Build history of the part. All positions in model axes, mm. Round coordinates to 2 decimals unless told otherwise and drop trailing zeros. Loops run counter-clockwise (first coordinate to the right, second up) from the corner with the lowest first, then second, coordinate; pieces in that order, holes last. Notation, with made-up numbers: M -23,89.25 L -4,89.25 A33 ccw -4,125.25 Z; hole C -9,-7.75 d10. An arc over 180 degrees is marked long. One line per item, written item: value.
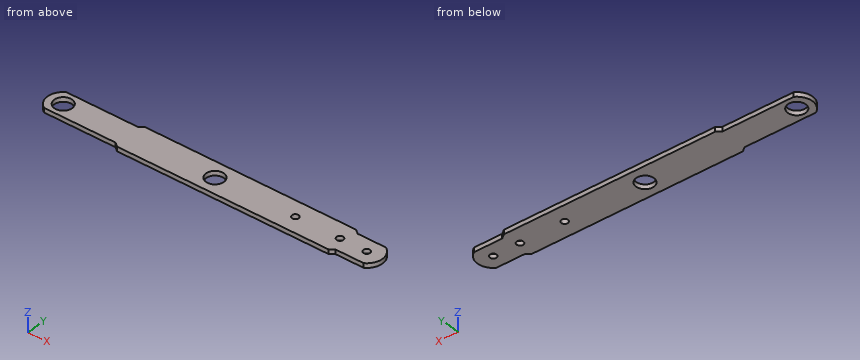
```python
from build123d import *

# Parameters (mm, degrees)
ESQUISSE1_R      = 1.5
ESQUISSE1_R_2    = 4
EXTRUSION1_DEPTH = 2


with BuildPart() as part:
    # Esquisse1 → Extrusion1 (new body)
    with BuildSketch(Plane.XY):
        with BuildLine():
            Line((71.605551275, 6), (59, 6))
            Line((59, 6), (57, 7.5))
            Line((57, 7.5), (-37.605551275, 7.5))
            Line((-37.605551275, 7.5), (-39.605551275, 6))
            Line((-39.605551275, 6), (-71.605551275, 6))
            ThreePointArc((-71.605551275, 6), (-75, 0), (-71.605551275, -6))
            Line((-71.605551275, -6), (-39.605551275, -6))
            Line((-39.605551275, -6), (-37.605551275, -7.5))
            Line((-37.605551275, -7.5), (57, -7.5))
            Line((57, -7.5), (59, -6))
            Line((59, -6), (71.605551275, -6))
            ThreePointArc((71.605551275, -6), (75, 0), (71.605551275, 6))
        make_face()
        with Locations((68, 0)):
            Circle(ESQUISSE1_R, mode=Mode.SUBTRACT)
        with Locations(Location((-68, 0, 0), (0, 0, 180))):
            Circle(ESQUISSE1_R_2, mode=Mode.SUBTRACT)
        Circle(ESQUISSE1_R_2, mode=Mode.SUBTRACT)
        with Locations((56, 0)):
            Circle(ESQUISSE1_R, mode=Mode.SUBTRACT)
        with Locations((36, 0)):
            Circle(ESQUISSE1_R, mode=Mode.SUBTRACT)
    extrude(amount=EXTRUSION1_DEPTH)


solid = part.part
```
Item 1: Drop flat-ended pins along their axis: P1, Ø3.5, axis at x = 68, y = 0, coming from the +Z side; P2, Ø1, axis at x = 67, z = 1.5, coming from the +Y side; P3, Ø5, axis at x = 0, y = 0, coming from the -Z side; P4, Ø0.6, axis at x = -51, z = 1.5, coming from the -Y side. Give the stop position or say it passes through.
Check values:
P1: stops at z = 2
P2: stops at y = 6
P3: passes through
P4: stops at y = -6
Item 2: Slice it at A-A, the plane x = 68. Give the cut face in (y, z).
Check values:
outline: M -6,0 L -1.5,0 L -1.5,2 L -6,2 Z; M 1.5,0 L 6,0 L 6,2 L 1.5,2 Z
Item 3: Slice it at B-B, the plane z = 0.3. Give the cut face in (x, y).
Check values:
outline: M -71.61,-6 L -39.61,-6 L -37.61,-7.5 L 57,-7.5 L 59,-6 L 71.61,-6 A7 ccw 71.61,6 L 59,6 L 57,7.5 L -37.61,7.5 L -39.61,6 L -71.61,6 A7 ccw Z; hole C -68,0 d8; hole C 0,0 d8; hole C 36,0 d3; hole C 56,0 d3; hole C 68,0 d3
Item 4: Wall check: line 1 along X through (y, z) = (-1, 1.95); line 2 along Y through (x, z) = (36, 1.65); line 3 along X through (y, z) = (0.5, 0.85). Give the ranges that are in metal, low to high.
Check values:
line 1: x = -74.93 to -71.87, -64.13 to -3.87, 3.87 to 34.88, 37.12 to 54.88, 57.12 to 66.88, 69.12 to 74.93
line 2: y = -7.5 to -1.5, 1.5 to 7.5
line 3: x = -74.98 to -71.97, -64.03 to -3.97, 3.97 to 34.59, 37.41 to 54.59, 57.41 to 66.59, 69.41 to 74.98
Item 5: Slice it at C-C, the plane x = -68. Give the cut face in (y, z).
Check values:
outline: M -6,0 L -4,0 L -4,2 L -6,2 Z; M 4,0 L 6,0 L 6,2 L 4,2 Z
